from build123d import *

# Parameters (mm, degrees)
SKETCH6_R                        = 66.04
BOSS_EXTRUDE1_DEPTH              = 2.54
PIPE_TAP_DRILL_FOR_1_4_TAP_GN2_D = 11.1252


with BuildPart() as part:
    # Sketch1 → Revolve1 (revolve)
    with BuildSketch(Plane.XY, mode=Mode.PRIVATE) as revolve1_sk:
        Polygon((0, 0), (72.898, 0), (72.898, 2.4638), (69.977, 2.4638), (69.977, 7.4422), (72.898, 7.4422), (72.898, 9.906), (66.548, 9.906), (66.548, 6.35), (0, 6.35), align=None)
    revolve(revolve1_sk.sketch.rotate(Axis((0, 48.192213231, 0), (0, -1, 0)), 180), axis=Axis((0, 48.192213231, 0), (0, -1, 0)))

    # Sketch6 → Boss-Extrude1 (add)
    with BuildSketch(Plane.XZ):
        Circle(SKETCH6_R)
    extrude(amount=BOSS_EXTRUDE1_DEPTH)

    # Pipe Tap Drill for 1/4 Tap - GN2 (through all)
    with Locations(Plane(origin=(0, 6.35, 0), x_dir=(1, 0, 0), z_dir=(0, 1, 0))):
        with Locations((0, 0)):
            Hole(PIPE_TAP_DRILL_FOR_1_4_TAP_GN2_D / 2)


solid = part.part
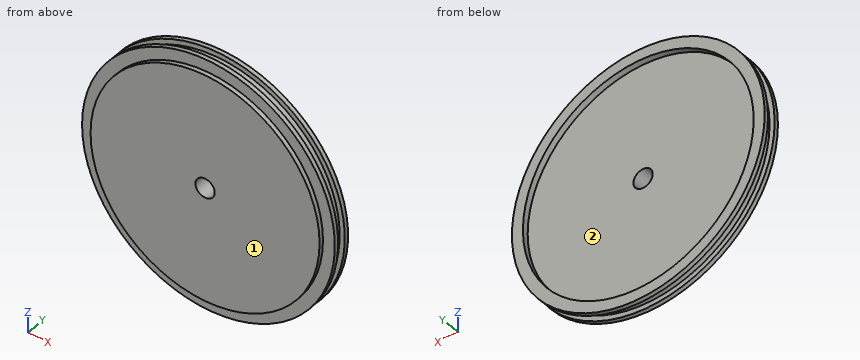
The listing builds one solid part. Answer for the finished solid, in the listing's coordinates (mm). Face numbers are marked on the shaded views. Give positions to 0.01 mm unless a question says otherwise; leave off trailing zeros. Write each loop counter-clockwise with the first axis right and the second up, starting at its lowest first coordinate (ties: lowest second). Pieces come first, ordered by that corner, then holes. Notation, with made-up numbers: (11.5, -15) - (57.5, -15) arc R21 cw to (57.5, 22) - close; hole circle Ø8 at (-16.5, 74). An arc over 180 degrees is marked (long way). One line per question, with ' | ' between items. Start each with the question number.
1. Section D-D, the plane z = 54 is taken. Determine the outline of the cut face in (x, y).
2. Straight lines are drawn through the part: line 1 (Z direction, x = 0, y = 0.75); line 2 (Z direction, x = 0, y = 8.9); line 3 (Y direction, x = -38, z = -23). For each, find the intervals that lie inside material, in ascending order.
3. Given P1, Ø1.5, axis at x = -24.5, z = -35, coming from the +Y side; P2, Ø6, axis at x = -12.5, y = 1, coming from the +Z side; P3, Ø1.5, axis at y = 2, z = 9.5, coming from the +X side; P4, Ø10, axis at x = 0, z = 0, coming from the -Y side, each flat-ended and moving along its own axis, determine where each tip first touches the part or whether it passes through.
4. Section C-C, the plane x = 40 is taken. Determine the outline of the cut face in (y, z), then the cut area to 3 significant figures.
5. Section B-B, the plane x = 0 is taken. Determine the outline of the cut face in (y, z), then the cut area to 3 significant figures.
6. Section A-A, the plane z = 0 is taken. Determine the outline of the cut face in (x, y).
7. Determine the mould class of the marked faces 1 and 2 for opening direction Z: +Z half, -Z half, draft (parallel to the pull), parting line (faces both ways), or undercut.
Result:
1) outline: (-48.97, 0) - (-38.02, 0) - (-38.02, -2.54) - (38.02, -2.54) - (38.02, 0) - (48.97, 0) - (48.97, 2.46) - (44.51, 2.46) - (44.51, 7.44) - (48.97, 7.44) - (48.97, 9.91) - (38.89, 9.91) - (38.89, 6.35) - (-38.89, 6.35) - (-38.89, 9.91) - (-48.97, 9.91) - (-48.97, 7.44) - (-44.51, 7.44) - (-44.51, 2.46) - (-48.97, 2.46) - close
2) line 1: z = -72.9 to -5.56, 5.56 to 72.9 | line 2: z = -72.9 to -66.55, 66.55 to 72.9 | line 3: y = -2.54 to 6.35
3) P1: stops at y = 6.35 | P2: stops at z = 72.28 | P3: stops at x = 72.37 | P4: passes through
4) outline: (-2.54, -52.55) - (0, -52.55) - (0, -60.94) - (2.46, -60.94) - (2.46, -57.42) - (7.44, -57.42) - (7.44, -60.94) - (9.91, -60.94) - (9.91, -53.18) - (6.35, -53.18) - (6.35, 53.18) - (9.91, 53.18) - (9.91, 60.94) - (7.44, 60.94) - (7.44, 57.42) - (2.46, 57.42) - (2.46, 60.94) - (0, 60.94) - (0, 52.55) - (-2.54, 52.55) - close | area: 1,060 mm2
5) outline: (-2.54, -66.04) - (0, -66.04) - (0, -72.9) - (2.46, -72.9) - (2.46, -69.98) - (7.44, -69.98) - (7.44, -72.9) - (9.91, -72.9) - (9.91, -66.55) - (6.35, -66.55) - (6.35, -5.56) - (-2.54, -5.56) - close; (-2.54, 5.56) - (6.35, 5.56) - (6.35, 66.55) - (9.91, 66.55) - (9.91, 72.9) - (7.44, 72.9) - (7.44, 69.98) - (2.46, 69.98) - (2.46, 72.9) - (0, 72.9) - (0, 66.04) - (-2.54, 66.04) - close | area: 1,180 mm2
6) outline: (-72.9, 0) - (-66.04, 0) - (-66.04, -2.54) - (-5.56, -2.54) - (-5.56, 6.35) - (-66.55, 6.35) - (-66.55, 9.91) - (-72.9, 9.91) - (-72.9, 7.44) - (-69.98, 7.44) - (-69.98, 2.46) - (-72.9, 2.46) - close; (5.56, -2.54) - (66.04, -2.54) - (66.04, 0) - (72.9, 0) - (72.9, 2.46) - (69.98, 2.46) - (69.98, 7.44) - (72.9, 7.44) - (72.9, 9.91) - (66.55, 9.91) - (66.55, 6.35) - (5.56, 6.35) - close
7) face 1: draft | face 2: undercut
